from build123d import *

# Parameters (mm, degrees)
BOSS_EXTRUDE1_DEPTH = 15
BOSS_EXTRUDE2_DEPTH = 15
FILLET4_R           = 0.8


with BuildPart() as part:
    # Sketch1 → Boss-Extrude1 (new, symmetric)
    with BuildSketch(Plane.XY):
        with BuildLine():
            Line((-13.329010746, 33.041463317), (120.837574837, 87.164606832))
            ThreePointArc((120.837574837, 87.164606832), (249.989705965, 0), (120.837574837, -87.164606832))
            Line((120.837574837, -87.164606832), (-13.329010746, -33.041463317))
            ThreePointArc((-13.329010746, -33.041463317), (-35.628651751, 0), (-13.329010746, 33.041463317))
        make_face()
        with BuildLine():
            Line((-12.505970238, 31.001217174), (121.660615345, 85.124360689))
            ThreePointArc((121.660615345, 85.124360689), (247.789705965, 0), (121.660615345, -85.124360689))
            Line((121.660615345, -85.124360689), (-12.505970238, -31.001217174))
            ThreePointArc((-12.505970238, -31.001217174), (-33.428651751, 0), (-12.505970238, 31.001217174))
        make_face(mode=Mode.SUBTRACT)
    extrude(amount=BOSS_EXTRUDE1_DEPTH, both=True)

    # Sketch2 → Boss-Extrude2 (add, symmetric)
    with BuildSketch(Plane.XY):
        with BuildLine():
            Line((26.425162942, 46.022572764), (26.179278266, 46.606945289))
            Line((26.179278266, 46.606945289), (30.962929341, 48.536682358))
            Line((30.962929341, 48.536682358), (31.237715226, 47.963968655))
            ThreePointArc((31.237715226, 47.963968655), (29.866253214, 44.428056099), (26.425162942, 46.022572764))
        make_face()
    extrude(amount=BOSS_EXTRUDE2_DEPTH, both=True)

    # Fillet4
    fillet4_edges = [part.edges().sort_by_distance(p)[0] for p in [
        (30.962929341, 48.536682358, 0),
        (26.179278266, 46.606945289, 0),
    ]]
    fillet(fillet4_edges, radius=FILLET4_R)


solid = part.part
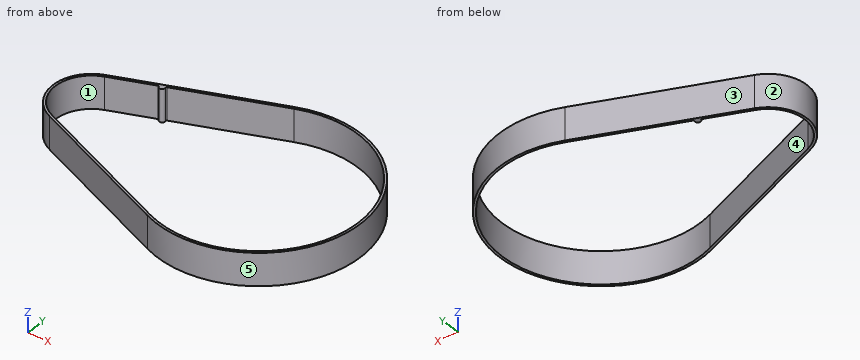
For this review, take the finished solid that the model builds, in its own axes (mm). Face numbers are marked on the shaded views. A direction names the side the tool comes from. Coordinates: 2 decimals unless noted, no trailing zeros. Loops run counter-clockwise (first coordinate to the right, second up) from the corner with the lowest first, then second, coordinate; pieces in that order, holes last. Notation, with made-up numbers: (-38, 65.5) - (-31, 65.5) arc R21 ccw to (-31, 93.5) - close; hole circle Ø8 at (60.5, 66). An arc over 180 degrees is marked (long way). Return JSON: item names as keys, results as strings.
Item 1: Take a section at B-B (x = 103). Give the boundary of the cut face in (y, z).
Determined:
{"outline": "(-79.97, -15) - (-77.6, -15) - (-77.6, 15) - (-79.97, 15) - close; (77.6, -15) - (79.97, -15) - (79.97, 15) - (77.6, 15) - close"}
Item 2: Insertion check: pin 1 (8 mm diameter, centred on y = 35, z = -5.5, fed in from -X); pin 2 (10 mm diameter, centred on x = 116, z = -1.5, fed in from -Y); pin 3 (12 mm diameter, centred on x = 3.5, z = 8.5, fed in from -Y). Each pin has a flat end and moves straight along its axis. Give the tip position at first contact, or say it passes through.
Determined:
{"pin 1": "stops at x = -17.56", "pin 2": "stops at y = -87.23", "pin 3": "stops at y = -42.25"}
Item 3: For the marked faces 1 and 2, list the 3-axis set-ups (+Z, -Z, +X, -X, +Y, -Y) from which the entire face can be reached by the end or side of a thin tool; tool diameter is ignored.
Determined:
{"face 1": "+Z, -Z", "face 2": "+Z, -Z, -X"}
Item 4: Take a section at A-A (y = 0). Give the boundary of the cut face in (x, z), then the cut area to 3 significant figures.
Determined:
{"outline": "(-35.63, -15) - (-33.43, -15) - (-33.43, 15) - (-35.63, 15) - close; (247.79, -15) - (249.99, -15) - (249.99, 15) - (247.79, 15) - close", "area": "132 mm2"}
Item 5: Mouldability with a two-part tool opening along Y and no side actions: class the marked faces 3, 4 and 5 as pulls with the +Y half, pulls with the -Y half, needs draft (parallel to the pull), parting line crosses it, or undercut.
Determined:
{"face 3": "pulls with the +Y half", "face 4": "undercut", "face 5": "parting line crosses it"}
Item 6: For line 1 (Y direction, x = 156, z = -3); line 2 (X direction, y = 0, z = -2); line 3 (X direction, y = 46, z = 0.5), list the stretches that pass through material, from the lowest coordinate up.
Determined:
{"line 1": "y = -93.99 to -91.79, 91.79 to 93.99", "line 2": "x = -35.63 to -33.43, 247.79 to 249.99", "line 3": "x = 18.79 to 24.67, 26.41 to 31.35, 235.43 to 237.96"}
